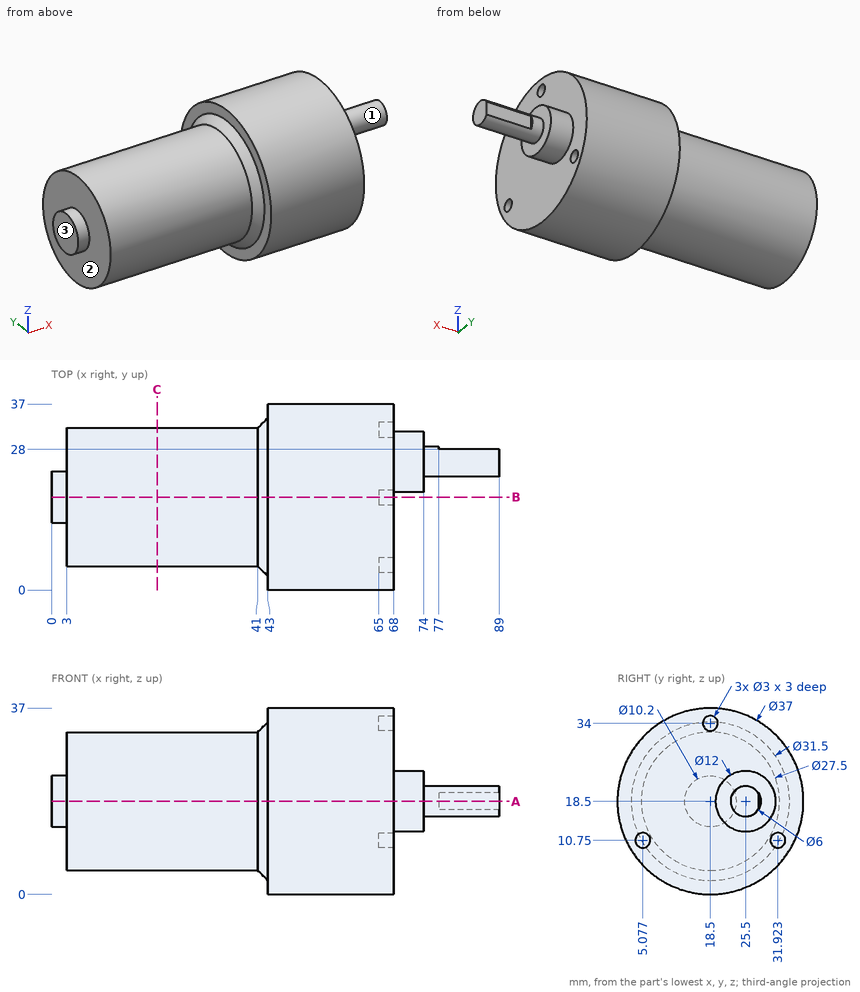
Print and shaded views of the part. All mm, measured from the part's lowest x, y and z. A direction names the side the tool comes from. Round coordinates to 2 decimals unless told otherwise and drop trailing zeros. Write each loop counter-clockwise with the first axis right and the second up, starting at its lowest first coordinate (ties: lowest second). Pieces come first, ordered by that corner, then holes. Notation, with made-up numbers: M -4.5,64 L 35.5,64 A34 ccw 35.5,96 Z; hole C -10,3.25 d5. An arc over 180 degrees is marked long. Use a Markdown table: item, result. Add a question column.
1. 3-axis set-ups, long thin cutter, end or side, ignore diameter. For the marked faces 1, 2 and 3: which of +Z, -Z, +X, -X, +Y, -Y reach the whole face in a straight line?
2. Flat gauge pins, fed straight in: P1, Ø5, axis at y = 26.5, z = 8, coming from the -X side; P2, Ø2.5, axis at y = 5, z = 11.5, coming from the +X side; P3, Ø10, axis at x = 69.5, y = 12, coming from the -Z side. Where does each tip first touch, or does it go through?
3. Slice it at A-A on z = 18.5. Give the cut face in (x, y), then the cut area to 3 significant figures.
4. Slice it at B-B on y = 18.5. Give the cut face in (x, z), then the cut area to 3 significant figures.
5. Slice it at C-C on x = 21. Give the cut face in (y, z).
6. Drill centre lines: probe 1 along Y at (x, z) = (67.4, 10.75); probe 2 along X at (y, z) = (6, 17.5); probe 3 along Y at (x, z) = (72, 19). Where is each one in solid material? Low to high.
Reply:
| question | item | result |
|---|---|---|
| 1 | face 1 | +X |
| 1 | face 2 | -X |
| 1 | face 3 | +Z, -Z, -X, +Y, -Y |
| 2 | P1 | stops at x = 3 |
| 2 | P2 | stops at x = 68 |
| 2 | P3 | stops at z = 0.08 |
| 3 | outline | M 0,13.4 L 3,13.4 L 3,4.75 L 41,4.75 L 43,2.75 L 43,0 L 68,0 L 68,19.5 L 74,19.5 L 74,22.5 L 89,22.5 L 89,28 L 77,28 L 77,28.5 L 74,28.5 L 74,31.5 L 68,31.5 L 68,37 L 43,37 L 43,34.25 L 41,32.25 L 3,32.25 L 3,23.6 L 0,23.6 Z |
| 3 | area | 2,220 mm^2 |
| 4 | outline | M 0,13.4 L 3,13.4 L 3,4.75 L 41,4.75 L 43,2.75 L 43,0 L 68,0 L 68,32.5 L 65,32.5 L 65,35.5 L 68,35.5 L 68,37 L 43,37 L 43,34.25 L 41,32.25 L 3,32.25 L 3,23.6 L 0,23.6 Z |
| 4 | area | 2,050 mm^2 |
| 5 | outline | C 18.5,18.5 d27.5 |
| 6 | probe 1 | y = 1.7 to 3.58, 6.58 to 30.42, 33.42 to 35.3 |
| 6 | probe 2 | x = 3 to 68 |
| 6 | probe 3 | y = 19.52 to 31.48 |
